Can you work these out from the model? Positions are in its coordinate system, mm. A direction names the side the tool comes from. Give positions to 0.01 mm unless a question says otherwise; leave off trailing zeros. Write each loop counter-clockwise with the first axis right and the second up, starting at its lowest first coordinate (ties: lowest second). Pieces come first, ordered by that corner, then holes. Notation, with made-up numbers: (-20.75, -35) - (8.25, -35) arc R28 cw to (8.25, -3) - close; hole circle Ø10 at (77, 42.25). An arc over 180 degrees is marked (long way). Use a Markdown table: item, result. Add a question column.
```python
from build123d import *

# Parameters (mm, degrees)
BOSS_EXTRUDE1_DEPTH = 86
SKETCH2_W           = 41
SKETCH2_H           = 2
BOSS_EXTRUDE2_DEPTH = 2
SKETCH3_W           = 38.84033909
SKETCH3_H           = 2
BOSS_EXTRUDE3_DEPTH = 0.25
FILLET2_R           = 0.5
FILLET1_R           = 3
CUT_EXTRUDE1_REACH  = 92.449
SKETCH4_R           = 2
FILLET3_R           = 0.5


with BuildPart() as part:
    # Sketch1 → Boss-Extrude1 (new body)
    with BuildSketch(Plane.XY):
        Polygon((18.194806353, 26), (19.420169545, 24.25), (-19.420169545, 24.25), (-18.194806353, 26), (-18.194806353, 26.1), (-20.5, 26.1), (-20.5, 28.1), (20.5, 28.1), (20.5, 26.1), (18.194806353, 26.1), align=None)
    extrude(amount=-BOSS_EXTRUDE1_DEPTH)

    # Sketch2 → Boss-Extrude2 (add)
    with BuildSketch(Plane(origin=(0, 0, -86), x_dir=(-1, 0, 0), z_dir=(0, 0, -1))):
        with Locations((0, 27.1)):
            Rectangle(SKETCH2_W, SKETCH2_H)
    extrude(amount=BOSS_EXTRUDE2_DEPTH)

    # Sketch3 → Boss-Extrude3 (add)
    with BuildSketch(Plane.XZ.offset(-24.25)):
        with Locations((0, -2.5)):
            Rectangle(SKETCH3_W, SKETCH3_H)
    extrude(amount=BOSS_EXTRUDE3_DEPTH)

    # Fillet2
    # the kernel refuses this fillet: 0.5 mm, written as the material it takes off along each edge
    with BuildSketch(Plane(origin=(-20.502701299, 24, -3.5), x_dir=(0, 1, 0), z_dir=(1, 0, 0)), Plane(origin=(20.502701299, 24, -1.5), x_dir=(0, 1, 0), z_dir=(-1, 0, 0))) as fillet2_piece_1:
        with BuildLine():
            CenterArc((0.5, 0.433012702), FILLET2_R, 180, 60)
            Line((0, 0.433012702), (-0.01, 0.433012702))
            Line((-0.01, 0.433012702), (-0.01, 0))
            Line((-0.01, 0), (0, -0.01))
            ThreePointArc((0, -0.01), (0.125, -0.01), (0.245, -0.008660254))
            Line((0.245, -0.008660254), (0.25, 0))
        make_face()
    extrude(amount=41.005402599, mode=Mode.SUBTRACT)

    # Fillet1
    fillet1_edges = [part.edges().sort_by_distance(p)[0] for p in [
        (-20.5, 27.1, 0),
        (20.5, 27.1, 0),
        (-20.5, 27.1, -88),
        (20.5, 27.1, -88),
    ]]
    fillet(fillet1_edges, radius=FILLET1_R)

    # Sketch4 → Cut-Extrude1 (cut, up to next)
    with BuildSketch(Plane(origin=(0, 28.1, 0), x_dir=(1, 0, 0), z_dir=(0, 1, 0)), mode=Mode.PRIVATE) as cut_extrude1_sk1:
        with Locations(Location((0, 73, 0), (0, 0, 270))):
            Circle(SKETCH4_R)
    cut_extrude1_tool1 = extrude(cut_extrude1_sk1.sketch, amount=-CUT_EXTRUDE1_REACH, mode=Mode.PRIVATE) & part.part
    # Sketch4 → Cut-Extrude1 (cut, up to next)
    with BuildSketch(Plane(origin=(0, 28.1, 0), x_dir=(1, 0, 0), z_dir=(0, 1, 0)), mode=Mode.PRIVATE) as cut_extrude1_sk2:
        with Locations((0, 15)):
            Circle(SKETCH4_R)
    cut_extrude1_tool2 = extrude(cut_extrude1_sk2.sketch, amount=-CUT_EXTRUDE1_REACH, mode=Mode.PRIVATE) & part.part
    add(cut_extrude1_tool1.solids().sort_by_distance((0, 28.1, -73))[0], mode=Mode.SUBTRACT)
    add(cut_extrude1_tool2.solids().sort_by_distance((0, 28.1, -15))[0], mode=Mode.SUBTRACT)

    # Fillet3
    fillet3_edges = [part.edges().sort_by_distance(p)[0] for p in [
        (20.5, 28.1, -44),
        (0, 28.1, 0),
        (19.621320344, 28.1, -0.878679656),
        (-19.621320344, 28.1, -0.878679656),
        (19.621320344, 28.1, -87.121320344),
        (-19.621320344, 28.1, -87.121320344),
        (-20.5, 28.1, -44),
        (0, 28.1, -88),
    ]]
    fillet(fillet3_edges, radius=FILLET3_R)


solid = part.part
```
Q1. If we mould it in two halves opening along X, with no side actions, what happens to faces 5 (the flat face through (20, 26.1, -54)), 6 (the cylindrical face through (19.64, 26.86, -87.1)), 7 (the cylindrical face through (0, 26, -17))? For each: released by +X, released by -X, zero draft, split by the parting line, or undercut.
Q2. On a 3-axis mill with a long thin cutter (end or side, diameter ignored), from which of +Z, -Z, +X, -X, +Y, -Y can I reach the whole of each face in a straight line? I mean faces 1 (the flat face through (18.799, 25.137, -42.439)), 2 (the flat face through (-18.82, 25.11, -42.44)), 3 (the flat face through (0, 24.25, -44)), 4 (the flat face through (0, 24.25, -1)). Say none if no direction works.
Q3. Suppose I cut it at C-C (x = 12). Please give me the cut outline in (y, z), and give its area (3 significant figures).
Q4. Suppose I cut it at B-B (z = -73). Please give me the cut outline in (x, y).
Q5. Suppose I cut it at D-D (z = -51). Please give me the cut outline in (x, y).
Q6. If I drill on probe 1 along X at (y, z) = (26.65, -15); probe 2 along Y at (x, z) = (8.5, -77); probe 3 along X at (y, z) = (25.25, -73.5), over which ranges is the centre line in solid material (lowest first)? Write a range as [from, to].
Q7. Suppose I cut it at A-A (x = 0). Please give me the cut outline in (y, z).
Q8. I'm going to push flat-ended pins straight in: P1, Ø3, axis at x = 0, z = -73, coming from the +Y side; P2, Ø2, axis at y = 24.5, z = -79, coming from the +X side; P3, Ø0.5, axis at x = -9.5, z = -1, coming from the -Y side; P4, Ø1.5, axis at x = 0, y = 24.5, coming from the -Z side. Where does each tip first touch, or does it pass through?
Derived:
| question | item | result |
|---|---|---|
| 1 | face 5 | zero draft |
| 1 | face 6 | released by +X |
| 1 | face 7 | undercut |
| 2 | face 1 | +Z, -Z, +X |
| 2 | face 2 | +Z, -Z, -X |
| 2 | face 3 | -Z, +X, -X, -Y |
| 2 | face 4 | +Z, +X, -X, -Y |
| 3 | outline | (24, -3.07) arc R0.5 ccw to (24.25, -3.5) - (24.25, -86) - (26.1, -86) - (26.1, -88) - (27.6, -88) arc R0.5 ccw to (28.1, -87.5) - (28.1, -0.5) arc R0.5 ccw to (27.6, 0) - (24.25, 0) - (24.25, -1.5) arc R0.5 ccw to (24, -1.93) - close |
| 3 | area | 335 mm² |
| 4 | outline | (-20.5, 26.1) - (-18.19, 26.1) - (-18.19, 26) - (-19.42, 24.25) - (-2, 24.25) - (-2, 28.1) - (-20, 28.1) arc R0.5 ccw to (-20.5, 27.6) - close; (2, 24.25) - (19.42, 24.25) - (18.19, 26) - (18.19, 26.1) - (20.5, 26.1) - (20.5, 27.6) arc R0.5 ccw to (20, 28.1) - (2, 28.1) - close |
| 5 | outline | (-20.5, 26.1) - (-18.19, 26.1) - (-18.19, 26) - (-19.42, 24.25) - (19.42, 24.25) - (18.19, 26) - (18.19, 26.1) - (20.5, 26.1) - (20.5, 27.6) arc R0.5 ccw to (20, 28.1) - (-20, 28.1) arc R0.5 ccw to (-20.5, 27.6) - close |
| 6 | probe 1 | [-20.5, -2], [2, 20.5] |
| 6 | probe 2 | [24.25, 28.1] |
| 6 | probe 3 | [-18.72, -1.94], [1.94, 18.72] |
| 7 | outline | (24, -3.07) arc R0.5 ccw to (24.25, -3.5) - (24.25, -13) - (28.1, -13) - (28.1, -0.5) arc R0.5 ccw to (27.6, 0) - (24.25, 0) - (24.25, -1.5) arc R0.5 ccw to (24, -1.93) - close; (24.25, -86) - (26.1, -86) - (26.1, -88) - (27.6, -88) arc R0.5 ccw to (28.1, -87.5) - (28.1, -75) - (24.25, -75) - close; (24.25, -71) - (28.1, -71) - (28.1, -17) - (24.25, -17) - close |
| 8 | P1 | through |
| 8 | P2 | x = 19.42 |
| 8 | P3 | y = 24.25 |
| 8 | P4 | z = -86 |
